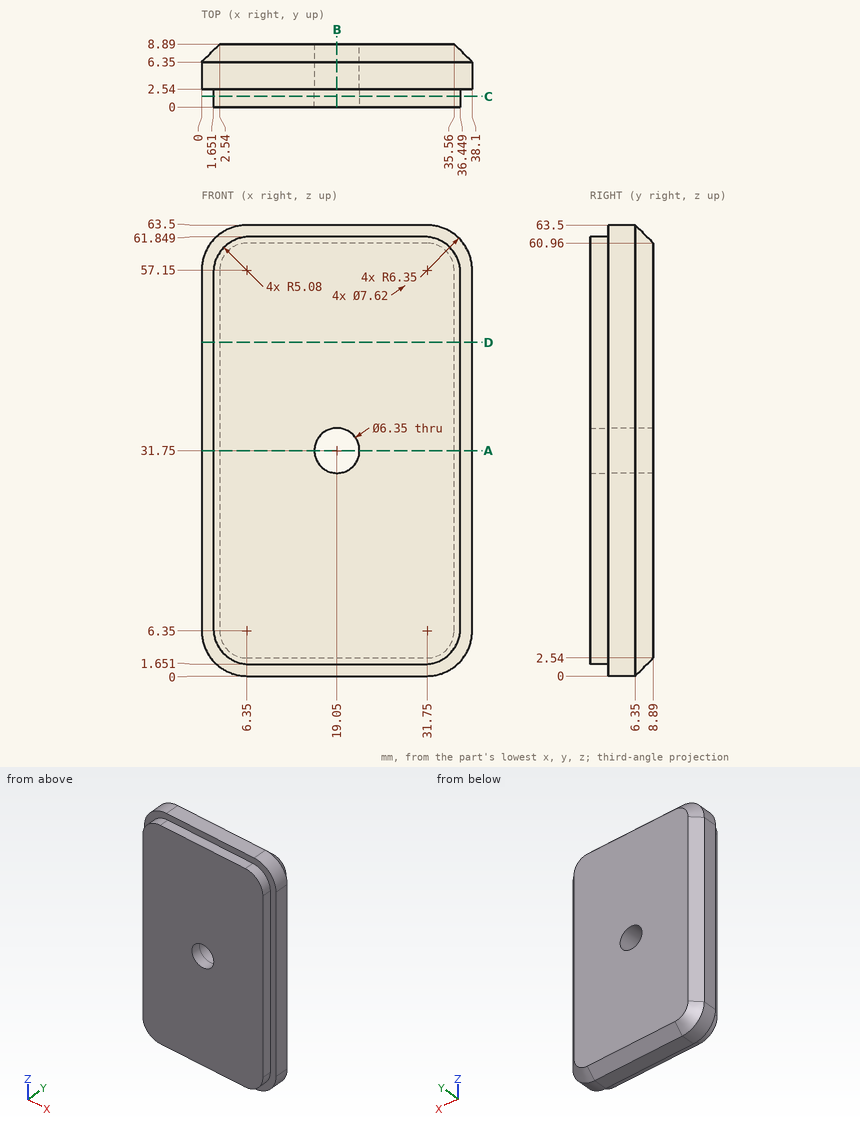
Source: three-view drawing plus pictorial views. Frame: mm from the lowest corner of the part. Give positions to 0.01 mm unless a question says otherwise; leave off trailing zeros. Order: outer loops, then holes, each group sorted by start corner. A loop starts at its lowest first (then second) coordinate and runs counter-clockwise, first axis right, second up. Notation, with made-up numbers: (17, 56.5) - (25, 56.5) arc R21 ccw to (25, 74.5) - close; hole circle Ø8 at (15.25, 57.5). An arc over 180 degrees is marked (long way). Put each result on its own line as item: value.
Item 1: Section query A-A, the plane z = 31.75. Return loops of the section in (x, y) (3 decimals).
Found:
outline: (0, 2.54) - (1.651, 2.54) - (1.651, 0) - (15.875, 0) - (15.875, 8.89) - (2.54, 8.89) - (0, 6.35) - close; (22.225, 0) - (36.449, 0) - (36.449, 2.54) - (38.1, 2.54) - (38.1, 6.35) - (35.56, 8.89) - (22.225, 8.89) - close
Item 2: Section query D-D, the plane z = 47. Return loops of the section in (x, y), then the cut area to 3 significant figures.
Found:
outline: (0, 2.54) - (1.65, 2.54) - (1.65, 0) - (36.45, 0) - (36.45, 2.54) - (38.1, 2.54) - (38.1, 6.35) - (35.56, 8.89) - (2.54, 8.89) - (0, 6.35) - close
area: 324 mm^2
Item 3: Ray query, L1, parallel to Z at x = 19.05, y = 2 (3 decimals); L2, parallel to X at y = 0.75, z = 37.5; L3, parallel to Z at x = 19.05, y = 4 (3 decimals). Return the intervals inside material, ascending. Write a range as from..to.
Found:
L1: z = 1.651..28.575, 34.925..61.849
L2: x = 1.65..36.45
L3: z = 0..28.575, 34.925..63.5
Item 4: Section query B-B, the plane x = 19.05. Return loops of the section in (y, z) (3 decimals).
Found:
outline: (0, 1.651) - (2.54, 1.651) - (2.54, 0) - (6.35, 0) - (8.89, 2.54) - (8.89, 28.575) - (0, 28.575) - close; (0, 34.925) - (8.89, 34.925) - (8.89, 60.96) - (6.35, 63.5) - (2.54, 63.5) - (2.54, 61.849) - (0, 61.849) - close
Item 5: Contact query for flat-ended pins moving along their axis: pin 1 (2 mm diameter, centred on x = 23.5, y = 1.5, fed in from +Z); pin 2 (3 mm diameter, centred on x = 21, y = 1, fed in from -Z); pin 3 (3 mm diameter, centred on y = 1, z = 39.5, fed in from +X). Output: stop coordinate, or through.
Found:
pin 1: stops at z = 61.85
pin 2: stops at z = 1.65
pin 3: stops at x = 36.45
Item 6: Section query C-C, the plane y = 1.5. Return loops of the section in (x, z) (3 decimals).
Found:
outline: (1.651, 6.731) arc R5.08 ccw to (6.731, 1.651) - (31.369, 1.651) arc R5.08 ccw to (36.449, 6.731) - (36.449, 56.769) arc R5.08 ccw to (31.369, 61.849) - (6.731, 61.849) arc R5.08 ccw to (1.651, 56.769) - close; hole circle Ø6.35 at (19.05, 31.75)
